Verification items for the finished model (mm, model axes). A direction names the side the tool comes from. Round coordinates to 2 decimals unless told otherwise and drop trailing zeros. Loops run counter-clockwise (first coordinate to the right, second up) from the corner with the lowest first, then second, coordinate; pieces in that order, holes last. Notation, with made-up numbers: (82, -0.75) -> (86, -0.75) arc R25 cw to (86, 24.25) -> close; hole circle Ø7 at (-23.75, 21.25). An arc over 180 degrees is marked (long way). Write item = value, one per line.
Autodesk Inventor part; units mm, degrees
ref_plane "YZ Plane" through (0, 0, 0) normal (1, 0, 0) x (0, 1, 0)
ref_plane "XZ Plane" through (0, 0, 0) normal (0, 1, 0) x (-1, 0, 0)
ref_plane "XY Plane" through (0, 0, 0) normal (0, 0, 1) x (1, 0, 0)
sketch "Sketch1" plane through (0, 0, 0) normal (0, 0, 1) x (1, 0, 0)
  line L0 (0, 0) -> (-56.9976, 0)
  line L1 (-56.9976, 0) -> (-56.9976, 38.1)
  line L2 (-56.9976, 38.1) -> (0, 38.1)
  line L3 (0, 38.1) -> (0, 0)
  line L4 (0, 38.1) -> (-7.493, 38.1)
  line L5 (-7.493, 38.1) -> (-7.493, 8.1026)
  line L6 (-56.9976, 38.1) -> (-49.5046, 38.1)
  line L7 (-49.5046, 38.1) -> (-49.5046, 8.1026)
  circle A0 centre (-49.5046, 8.1026) radius 3.302
  circle A1 centre (-7.493, 8.1026) radius 3.302
  dimension "d1" = 56.9976
  dimension "d2" = 38.1
  dimension "d3" = 7.493
  dimension "d4" = 29.9974
  dimension "d5" = 7.493
  dimension "d6" = 6.604
  dimension "d7" = 6.604
extrude "Plate1" add sketch "Sketch1" along normal blind 3.175
sketch "Sketch2" plane through (0, 47.625, -9.525) normal (0, 1, 0) x (-1, 0, 0)
  line L0 (56.9976, 0) -> (0, 0)
  line L1 (0, 0) -> (0, -12.7)
  line L2 (0, -12.7) -> (56.9976, -12.7)
  line L3 (56.9976, -12.7) -> (56.9976, 0)
edge flange "Flange1" height 25.4 angle 90 thickness 3.175 bend radius 9.525 thickness toward (0, 1, 0) relief tear relief width 3.175 relief depth 1.5875 edges at (-53.2511, 38.1, 0) wall of the first edge with corners at (-56.9976, 47.625, -9.525) (0, 47.625, -9.525) (0, 47.625, -22.225) (-56.9976, 47.625, -22.225)
bend "Bend1"
corner "Corner1"
sketch "Sketch3" plane through (-56.9976, 50.8, -22.225) normal (0, 1, 0) x (1, 0, 0)
  line L0 (0, -12.7) -> (56.9976, -12.7)
  line L1 (56.9976, 0) -> (56.9976, -12.7)
  line L2 (0, 0) -> (56.9976, 0)
  line L3 (0, -12.7) -> (0, 0)
  point P0 (56.9976, -22.225)
sketch "Sketch4" plane through (-56.9976, 50.8, -22.225) normal (0, 1, 0) x (1, 0, 0)
  line L0 (0, -12.7) -> (56.9976, -12.7)
  line L1 (56.9976, 0) -> (56.9976, -12.7)
  line L2 (0, 0) -> (56.9976, 0)
  line L3 (0, -12.7) -> (0, 0)
  point P0 (56.9976, -22.225)
sketch "Sketch5" plane through (-56.9976, 50.8, -22.225) normal (0, 1, 0) x (1, 0, 0)
  line L0 (0, -12.7) -> (56.9976, -12.7)
  line L1 (56.9976, 0) -> (56.9976, -12.7)
  line L2 (0, 0) -> (56.9976, 0)
  line L3 (0, -12.7) -> (0, 0)
  point P0 (56.9976, -22.225)
sketch "Sketch6" plane through (-56.9976, 50.8, -22.225) normal (0, 1, 0) x (1, 0, 0)
  line L0 (0, -12.7) -> (56.9976, -12.7)
  line L1 (56.9976, 0) -> (56.9976, -12.7)
  line L2 (0, 0) -> (56.9976, 0)
  line L3 (0, -12.7) -> (0, 0)
  point P0 (56.9976, -22.225)
equation "\"d9\" = BendReliefWidth"
equation "\"d10\" = BendReliefDepth"
equation "\"d11\" = MinimumRemnant"
equation "\"d12\" = BendRadius"
equation "\"d16\" = CornerReliefSize"
equation "\"d17\" = GapSize"
equation "\"d18\" = JacobiRadiusSize"
equation "\"BendRadius\" = Thickness"
equation "\"BendReliefWidth\" = Thickness"
equation "\"BendReliefDepth\" = 0.5 * Thickness"
equation "\"CornerReliefSize\" = 4 * Thickness"
equation "\"MinimumRemnant\" = 2 * Thickness"
equation "\"TransitionRadius\" = BendRadius"
equation "\"JacobiRadiusSize\" = BendRadius"
equation "\"GapSize\" = Thickness"
equation "\"d8\" = BendRadius"
properties part number "endstop"
(1) Sectioned sample at B-B, the plane x = -20. Record the cut outline in (y, z) (3 decimals).
Filled sheet:
outline = (0, 0) -> (38.1, 0) arc R9.525 cw to (47.625, -9.525) -> (47.625, -22.225) -> (50.8, -22.225) -> (50.8, -9.525) arc R12.7 ccw to (38.1, 3.175) -> (0, 3.175) -> close
(2) Sectioned sample at A-A, the plane x = -52. Record the cut outline in (y, z) (3 decimals).
Filled sheet:
outline = (0, 0) -> (5.94, 0) -> (5.94, 3.175) -> (0, 3.175) -> close; (10.265, 0) -> (38.1, 0) arc R9.525 cw to (47.625, -9.525) -> (47.625, -22.225) -> (50.8, -22.225) -> (50.8, -9.525) arc R12.7 ccw to (38.1, 3.175) -> (10.265, 3.175) -> close
(3) Draft check along X on faces 3 (the face through (0, 33, 1)), 4 (the face through (-4.443, 9.367, 1.565)), 5 (the face through (-28, 0, 2)). Enter one of: released by +X, released by -X, zero draft, split by the parting line, or undercut.
Filled sheet:
face_3 = released by +X
face_4 = undercut
face_5 = zero draft
(4) Material ranges on probe 1 along Y at (x, z) = (-14, -12) (3 decimals); probe 2 along Z at (x, y) = (-46.5, 2.5) (3 decimals); probe 3 along Y at (x, z) = (-26.5, -5.75) (3 decimals), recorded low to high. Write a range as from..to.
Filled sheet:
probe_1 = 47.625..50.8
probe_2 = 0..3.175
probe_3 = 46.845..50.226
(5) Set-up check for faces 1 (the face through (-28, 50.8, -16)), 2 (the face through (-28, 47.625, -16)): record each of +Z, -Z, +X, -X, +Y, -Y from which the full face is reachable in a straight line by a thin tool's end or side.
Filled sheet:
face_1 = +Z, -Z, +X, -X, +Y
face_2 = -Z, +X, -X, -Y
(6) Sectioned sample at D-D, the plane y = 33. Record the cut outline in (x, z) (3 decimals).
Filled sheet:
outline = (-56.998, 0) -> (0, 0) -> (0, 3.175) -> (-56.998, 3.175) -> close
(7) Go/stop test with flat-tipped pins: pin 1 Ø1.5 at (x, y) = (-46.5, 44) entering from -Z; pin 2 Ø6.5 at (x, z) = (-26, -17.5) entering from -Y (3 decimals); pin 3 Ø11.5 at (x, y) = (-16, 20.5) entering from -Z. Record where each tip stops, or that it passes through.
Filled sheet:
pin_1 = -2.71
pin_2 = 47.625
pin_3 = 0
(8) Sectioned sample at C-C, the plane z = 1. Record the cut outline in (x, y), and give its area (3 significant figures).
Filled sheet:
outline = (-57, 0) -> (0, 0) -> (0, 45.21) -> (-57, 45.21) -> close; hole circle Ø6.6 at (-49.5, 8.1); hole circle Ø6.6 at (-7.49, 8.1)
area = 2,510 mm2
